For this review, take the finished solid that the model builds, in its own axes (mm). A direction names the side the tool comes from. Coordinates: 2 decimals unless noted, no trailing zeros. Order: outer loops, then holes, each group sorted by start corner. A loop starts at its lowest first (then second) coordinate and runs counter-clockwise, first axis right, second up. Notation, with made-up numbers: (50, -5) - (105, -5) arc R17 ccw to (105, -1) - close; hole circle Ø7 at (80.25, 23.25). An arc over 180 degrees is marked (long way). One line per item, written item: value. Start each with the question number.
(1) Consider section D-D on z = 436.5. Write out the cut boundary in (x, y), then the cut area to 3 significant figures.
(2) Consider section C-C on y = 107.5. Write out the cut boundary in (x, z).
(3) To check wall thickness, follow line 1 along Y through (x, z) = (3, 56.5); line 2 along X through (y, z) = (162.5, 944); line 3 along Z through (x, y) = (20, 21). State the ranges of each line that lie inside material, in increasing order.
(4) Mouldability with a two-part tool opening along X and no side actions: class faces 4 (the flat face through (2, -81, 875)), 5 (the flat face through (-38, -18, 190)), 6 (the flat face through (1, -41, 117)) as released by +X, released by -X, zero draft, split by the parting line, or undercut.
(5) Consider section B-B on z = 209.5. Write out the cut boundary in (x, y).
(6) Clearance check with flat-ended pins moving along their axes: pin 1 (4 mm diameter, centred on x = -39.5, z = 157, fed in from +Y); pin 2 (5.5 mm diameter, centred on x = -5, z = 925, fed in from +Y); pin 3 (1.5 mm diameter, centred on x = 31.5, z = 142.5, fed in from +Y); pin 4 (4 mm diameter, centred on x = 2, y = -25.5, fed in from -Z). State where each tip first meets the part, or that it passes through.
(7) Consider section A-A on z = 939. Write out the cut boundary in (x, y).
(8) For faces 1 (the flat face through (-2, -81, 875)), 2 (the flat face through (2, 99, 906)), 3 (the flat face through (7, -53, 879)), list the 3-axis set-ups (+Z, -Z, +X, -X, +Y, -Y) from which the entire face can be reached by the end or side of a thin tool; tool diameter is ignored.
```python
from build123d import *

# Parameters (mm, degrees)
P_IDAT_VYSUNUT_M1_DEPTH      = 145
P_IDAT_VYSUNUT_M2_DEPTH      = 92
SKICA3_R                     = 27.5
P_IDAT_VYSUNUT_M3_DEPTH      = 60
P_IDAT_VYSUNUT_M4_DEPTH      = 500
P_IDAT_VYSUNUT_M4_DEPTH_BACK = 40
SKICA4_R                     = 8
P_IDAT_VYSUNUT_M5_DEPTH      = 2
P_IDAT_VYSUNUT_M5_DEPTH_BACK = 2
SKICA6_W                     = 280
SKICA6_H                     = 22
P_IDAT_VYSUNUT_M6_DEPTH      = 5


with BuildPart() as part:
    # Skica1 → Přidat vysunutím1 (new body)
    with BuildSketch(Plane.XY):
        with BuildLine():
            Line((-41.5, 0), (-41.5, -41))
            Line((-41.5, -41), (41.5, -41))
            Line((41.5, -41), (41.5, 0))
            Line((41.5, 0), (40, 0))
            ThreePointArc((40, 0), (0, 40), (-40, 0))
            Line((-40, 0), (-41.5, 0))
        make_face()
    extrude(amount=P_IDAT_VYSUNUT_M1_DEPTH)

    # Skica2 → Přidat vysunutím2 (add)
    with BuildSketch(Plane.XY.offset(145)):
        Polygon((-41.5, 0), (-38, 0), (-38, -37.5), (38, -37.5), (38, 0), (41.5, 0), (41.5, -41), (-41.5, -41), align=None)
    extrude(amount=P_IDAT_VYSUNUT_M2_DEPTH)

    # Skica3 → Přidat vysunutím3 (add)
    with BuildSketch(Plane.XZ.offset(41)):
        with Locations(Location((0, 209.5, 0), (0, 0, 90))):
            Circle(SKICA3_R)
    extrude(amount=P_IDAT_VYSUNUT_M3_DEPTH)

    # Skica4 → Přidat vysunutím4 (add, two sides: drawn at the far end of the back side and taken through both)
    with BuildSketch(Plane.XY.offset(237).offset(-P_IDAT_VYSUNUT_M4_DEPTH_BACK)):
        with Locations((0, -53)):
            Circle(SKICA4_R)
    extrude(amount=P_IDAT_VYSUNUT_M4_DEPTH + P_IDAT_VYSUNUT_M4_DEPTH_BACK)

    # Skica5 → Přidat vysunutím5 (add, two sides: drawn at the far end of the back side and taken through both)
    with BuildSketch(Plane(origin=(0, 0, 0), x_dir=(0, 0, -1), z_dir=(1, 0, 0)).offset(-P_IDAT_VYSUNUT_M5_DEPTH_BACK)):
        Polygon((-737, 1), (-737, -99), (-1017, -99), (-1017, 236), (-867, 236), align=None)
    extrude(amount=P_IDAT_VYSUNUT_M5_DEPTH + P_IDAT_VYSUNUT_M5_DEPTH_BACK)

    # Skica6 → Přidat vysunutím6 (add)
    with BuildSketch(Plane(origin=(2, 0, 0), x_dir=(0, 0, -1), z_dir=(1, 0, 0))):
        with Locations((-877, -53)):
            Rectangle(SKICA6_W, SKICA6_H)
    p_idat_vysunut_m6 = extrude(amount=P_IDAT_VYSUNUT_M6_DEPTH)

    # Zrcadlit1: Přidat vysunutím6 across plane
    add(p_idat_vysunut_m6.mirror(Plane(origin=(0, 0, 0), x_dir=(0, 0, 1), z_dir=(1, 0, 0))))


solid = part.part
```
Geometry check:
1. outline: circle Ø16 at (0, -53)
1. area: 201 mm^2
2. outline: (-2, 795.91) - (2, 795.91) - (2, 1017) - (-2, 1017) - close
3. line 1: y = -41 to 39.89
3. line 2: x = -2 to 2
3. line 3: z = 0 to 145
4. face 4: released by +X
4. face 5: undercut
4. face 6: zero draft
5. outline: (-41.5, -41) - (-27.5, -41) - (-27.5, -101) - (27.5, -101) - (27.5, -41) - (41.5, -41) - (41.5, 0) - (38, 0) - (38, -37.5) - (-38, -37.5) - (-38, 0) - (-41.5, 0) - close
6. pin 1: stops at y = 0
6. pin 2: stops at y = -42
6. pin 3: stops at y = 25.58
6. pin 4: stops at z = 0
7. outline: (-7, -64) - (-2, -64) - (-2, -99) - (2, -99) - (2, -64) - (7, -64) - (7, -42) - (2, -42) - (2, 236) - (-2, 236) - (-2, -42) - (-7, -42) - close
8. face 1: +Z, -X, -Y
8. face 2: +Z, +X, +Y
8. face 3: +Z, +X, +Y, -Y
